Read the model definition and answer for the solid it produces. Units are mm, in the model's axes. Coordinates: 2 decimals unless noted, no trailing zeros. Order: outer loops, then holes, each group sorted by start corner. A loop starts at its lowest first (then second) coordinate and runs counter-clockwise, first axis right, second up. Notation, with made-up numbers: M 0,-12.5 L 32,-12.5 A29 cw 32,26.5 Z; hole C 85,-2.5 d7. An arc over 180 degrees is marked long. One line per question, with ' | ' between items. Start each with the question number.
1) Find section A-A, the plane x = 0. Write down the section's boundary in (y, z).
2) Consider probe 1 along Y at (x, z) = (39, 7.5); probe 2 along Y at (x, z) = (0, 7.5); probe 3 along Z at (x, y) = (-22.5, 0). Determine where each line is inside the solid, lowest interval first.
3) Find section C-C, the plane y = 0. Count the separate pieces of the cut face and the enclosed holes in it, plus the area to 4 significant figures.
4) Find section B-B, the plane x = -17. Write down the section's boundary in (y, z), plus the area to 3 significant figures.
5) The mould has two halves that part along Z. Classify faces 1 (the face through (-1, 14, 15)), 2 (the face through (-29.885, 2.688, 11.716)), 3 (the face through (-12, 9, 0)), 4 (the face through (1, -20, 7)): +Z half, -Z half, draft (parallel to the pull), parting line (faces both ways), or undercut.
6) Given P1, Ø1.5, axis at y = 4, z = 4, coming from the -X side, flat-ended and moving along its own axis, determine where the tip first touches the part or whether it passes through.
from build123d import *

# Parameters (mm, degrees)
SKETCH_R          = 13.25
PAD_DEPTH         = 15
SKETCH001_R       = 5
POCKET_DEPTH      = 35.001
POCKET_DEPTH_BACK = -63.001
CHAMFER_SIZE      = 1
CHAMFER001_SIZE   = 1
CHAMFER002_SIZE   = 1


with BuildPart() as part:
    # Sketch → Pad (new body)
    with BuildSketch(Plane.XY):
        with BuildLine():
            ThreePointArc((-44.732538, 20), (-49, 0), (-44.732538, -20))
            Line((44.732538, -20), (-44.732538, -20))
            ThreePointArc((44.732538, -20), (49, 0), (44.732538, 20))
            Line((-44.732538, 20), (44.732538, 20))
        make_face()
        Circle(SKETCH_R, mode=Mode.SUBTRACT)
    extrude(amount=PAD_DEPTH)

    # Sketch001 → Pocket (cut, two sides)
    with BuildSketch(Plane.YZ.offset(-14)) as pocket_sk:
        with Locations((0, 7.5)):
            Circle(SKETCH001_R)
    extrude(amount=-POCKET_DEPTH, mode=Mode.SUBTRACT)
    extrude(pocket_sk.sketch, amount=-POCKET_DEPTH_BACK, mode=Mode.SUBTRACT)

    # Chamfer
    chamfer_edges = [part.edges().sort_by_distance(p)[0] for p in [
        (-13.25, 0, 0),
    ]]
    chamfer(chamfer_edges, length=CHAMFER_SIZE)

    # Chamfer001
    chamfer001_edges = [part.edges().sort_by_distance(p)[0] for p in [
        (-48.74423, -5, 7.5),
    ]]
    chamfer(chamfer001_edges, length=CHAMFER001_SIZE)

    # Chamfer002
    chamfer002_edges = [part.edges().sort_by_distance(p)[0] for p in [
        (48.74423, -5, 7.5),
    ]]
    chamfer(chamfer002_edges, length=CHAMFER002_SIZE)


solid = part.part
Report:
1) outline: M -20,0 L -14.25,0 L -13.25,1 L -13.25,15 L -20,15 Z; M 13.25,1 L 14.25,0 L 20,0 L 20,15 L 13.25,15 Z
2) probe 1: y = -20 to -5, 5 to 20 | probe 2: y = -20 to -13.25, 13.25 to 20 | probe 3: z = 0 to 2.5, 12.5 to 15
3) separate pieces: 4 | enclosed holes: 0 | area: 354.5 mm^2
4) outline: M -20,0 L 20,0 L 20,15 L -20,15 Z; hole C 0,7.5 d10 | area: 521 mm^2
5) face 1: +Z half | face 2: undercut | face 3: -Z half | face 4: draft
6) P1: stops at x = -48.81
